```python
from build123d import *

# Parameters (mm, degrees)
SKETCH_W     = 32
SKETCH_H     = 5
PAD_DEPTH    = 12
SKETCH001_R  = 3
HOLE_DEPTH   = 15.001
SKETCH002_W  = 32
SKETCH002_H  = 5
PAD001_DEPTH = 70


with BuildPart() as part:
    # Sketch → Pad (new body)
    with BuildSketch(Plane.XY):
        Polygon((-20, -10), (5, -10), (5, 0), (0, 0), (0, -7), (-20, -7), align=None)
        with Locations((16, 2.5)):
            Rectangle(SKETCH_W, SKETCH_H)
    extrude(amount=PAD_DEPTH)

    # Sketch001 (on Face1 of Pad) → Hole (cut, through all)
    with BuildSketch(Plane.XZ.offset(10)):
        with Locations((-7, 6)):
            Circle(SKETCH001_R)
    extrude(amount=-HOLE_DEPTH, mode=Mode.SUBTRACT)

    # Sketch002 → Pad001 (join)
    with BuildSketch(Plane.XY):
        with Locations((16, 2.5)):
            Rectangle(SKETCH002_W, SKETCH002_H)
    extrude(amount=PAD001_DEPTH)


solid = part.part
```
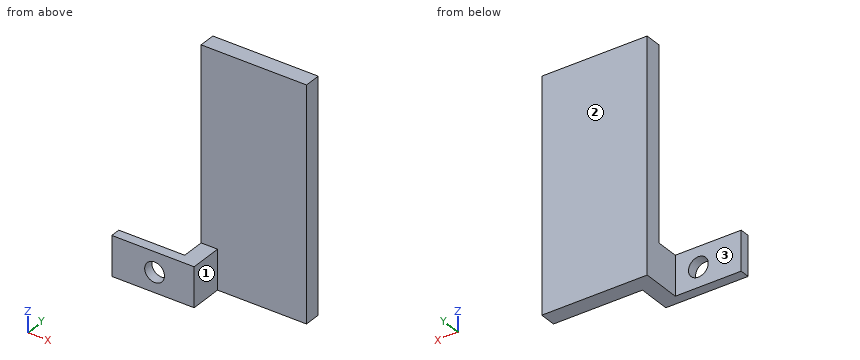
Here's how the part is built. I have some questions about the finished solid (model axes, mm). Face numbers are marked on the shaded views. A direction names the side the tool comes from. Coordinates: 2 decimals unless noted, no trailing zeros. Order: outer loops, then holes, each group sorted by start corner. A loop starts at its lowest first (then second) coordinate and runs counter-clockwise, first axis right, second up.
1) Will these pins go through, and if not, where does the flat tip stop? pin 1 (5 mm diameter, centred on x = 3, y = -0.5, fed in from -Z); pin 2 (4 mm diameter, centred on x = 22, z = 9.5, fed in from -Y); pin 3 (1 mm diameter, centred on y = 0.5, z = 56, fed in from -X); pin 4 (5 mm diameter, centred on y = -5, z = 9, fed in from +X).
2) I need wall thicknesses on line 1 (Z direction, x = -7, y = -8.25); line 2 (Y direction, x = 21.5, z = 42). Which ranges of each line are inside material? Lowest first, please.
3) Which directions (+Z, -Z, +X, -X, +Y, -Y) give clear straight access to the entire face, cutting with the end or side of a thin tool? Please do the marked faces 1, 2 and 3.
4) Imagine slicing it at A-A on z = 6. List the corners of the cut face in (x, y) for me, and give its area (3 significant figures).
5) Imagine slicing it at C-C on y = -7.75. List the corners of the cut face in (x, z) for me, and give its area (3 significant figures).
6) Imagine slicing it at D-D on z = 22.5. List the corners of the cut face in (x, y) for me.
7) Imagine slicing it at B-B on x = -7. List the corners of the cut face in (y, z) for me.
Response values:
1. pin 1: stops at z = 0
1. pin 2: stops at y = 0
1. pin 3: stops at x = 0
1. pin 4: stops at x = 5
2. line 1: z = 0 to 3, 9 to 12
2. line 2: y = 0 to 5
3. face 1: +Z, -Z, +X, -Y
3. face 2: +Z, -Z, +X, -X, +Y
3. face 3: +Z, -Z, -X, +Y
4. outline: (-20, -10) - (-10, -10) - (-10, -7) - (-20, -7) - close; (-4, -10) - (5, -10) - (5, 0) - (32, 0) - (32, 5) - (0, 5) - (0, -7) - (-4, -7) - close
4. area: 252 mm2
5. outline: (-20, 0) - (5, 0) - (5, 12) - (-20, 12) - close; hole circle Ø6 at (-7, 6)
5. area: 272 mm2
6. outline: (0, 0) - (32, 0) - (32, 5) - (0, 5) - close
7. outline: (-10, 0) - (-7, 0) - (-7, 3) - (-10, 3) - close; (-10, 9) - (-7, 9) - (-7, 12) - (-10, 12) - close
